Part model, mm, in its own coordinate system. A direction names the side the tool comes from. Give positions to 0.01 mm unless a question says otherwise; leave off trailing zeros. Write each loop counter-clockwise with the first axis right and the second up, starting at its lowest first coordinate (ties: lowest second). Pieces come first, ordered by that corner, then holes. Notation, with made-up numbers: M 53,29.5 L 101,29.5 A26 ccw 101,51.5 Z; hole C 42.25,-15.5 d9. An arc over 180 degrees is marked long. Answer as CSV lines item,"result". Start each with the question number.
1) Slice it at B-B, the plane x = 7.25. Give the cut face in (y, z), plus the area to 3 significant figures.
2) Wall check: line 1 along X through (y, z) = (-0.5, 5.5); line 2 along Y through (x, z) = (-3, 2.45); line 3 along Y through (x, z) = (7, 0.75). Give the ranges that are in metal, low to high. Write a range as from..to.
3) Slice it at A-A, the plane z = 24.5. Give the cut face in (x, y), plus the area to 3 significant figures.
4) Slice it at D-D, the plane y = 0. Give the number of separate pieces and of enclosed holes in the cut face, plus the area to 3 significant figures.
5) Pin check, flat tips, straight feed: pin 1 Ø11.5 at (x, y) = (-2, 2.5) entering from +Z; pin 2 Ø1 at (y, z) = (5.5, 25) entering from -X; pin 3 Ø10 at (x, z) = (-6, 29) entering from -Y. Stop position of each tip, or through.
6) Tool access for faces 1 (the cylindrical face through (6.25, 3.03, 1.52)), 2 (the cylindrical face through (11.7, 0.1, 14.5)): list every direction of +Z, -Z, +X, -X, +Y, -Y with a clear straight run to the whole face (end or side of a thin tool).
7) Mould opens along Y. For faces 3 (the cylindrical face through (12.06, -2.22, 16.85)), 4 (the flat face through (-12, 0, 33)) say: pulls with the +Y half, pulls with the -Y half, needs draft (parallel to the pull), parting line crosses it, or undercut.
8) Slice it at C-C, the plane x = 0. Give the cut face in (y, z), plus the area to 3 significant figures.
```python
from build123d import *
from build123d.topology import SkipClean

# Parameters (mm, degrees)
SKETCH1_R                           = 12.7
BOSS_EXTRUDE1_DEPTH                 = 3
SKETCH2_R                           = 0.75
CUT_EXTRUDE1_DEPTH                  = 3
BOSS_EXTRUDE2_DEPTH                 = 30
CUT_EXTRUDE2_REACH                  = 39.571
CUT_EXTRUDE2_END_RADIUS             = 12.7
SKETCH4_R                           = 2.5
CUT_EXTRUDE2_DIRECTION_2_REACH      = 39.571
CUT_EXTRUDE2_DIRECTION_2_END_RADIUS = 12.7


with BuildPart() as part:
    # Sketch1 → Boss-Extrude1 (new body)
    with BuildSketch(Plane.XY):
        Circle(SKETCH1_R)
    extrude(amount=BOSS_EXTRUDE1_DEPTH)

    # Sketch2 → Cut-Extrude1 (cut)
    with BuildSketch(Plane.XY.offset(3)):
        with Locations((0, 7)):
            Circle(SKETCH2_R)
        with Locations((-3, 7)):
            Circle(SKETCH2_R)
        with Locations((3, 7)):
            Circle(SKETCH2_R)
        with Locations((7, -3)):
            Circle(SKETCH2_R)
        with Locations((7, 0)):
            Circle(SKETCH2_R)
        with Locations((7, 3)):
            Circle(SKETCH2_R)
        with Locations((-3, -7)):
            Circle(SKETCH2_R)
        with Locations((0, -7)):
            Circle(SKETCH2_R)
        with Locations((3, -7)):
            Circle(SKETCH2_R)
        with Locations((-7, 3)):
            Circle(SKETCH2_R)
        with Locations((-7, 0)):
            Circle(SKETCH2_R)
        with Locations((-7, -3)):
            Circle(SKETCH2_R)
    extrude(amount=-CUT_EXTRUDE1_DEPTH, mode=Mode.SUBTRACT)

    # Sketch3 → Boss-Extrude2 (add)
    with SkipClean():  # the faces are left unmerged after this step: merging them gives an invalid solid
        with BuildSketch(Plane.XY.offset(3)):
            with BuildLine():
                Line((-8.980256121, 8.980256121), (-8.273149436, 8.273149436))
                ThreePointArc((-8.273149436, 8.273149436), (-11.700000136, 0), (-8.27314937, -8.27314937))
                Line((-8.27314937, -8.27314937), (-8.980256121, -8.980256121))
                ThreePointArc((-8.980256121, -8.980256121), (-12.7, 0), (-8.980256121, 8.980256121))
            make_face()
            with BuildLine():
                Line((8.980256121, 8.980256121), (8.273149436, 8.273149436))
                ThreePointArc((8.273149436, 8.273149436), (11.700000136, 0), (8.27314937, -8.27314937))
                Line((8.27314937, -8.27314937), (8.980256121, -8.980256121))
                ThreePointArc((8.980256121, -8.980256121), (12.7, 0), (8.980256121, 8.980256121))
            make_face()
        extrude(amount=BOSS_EXTRUDE2_DEPTH)

    # Cut-Extrude2: up to this cylinder (the profile starts inside it)
    with SkipClean():  # the faces are left unmerged after this step: merging them gives an invalid solid
        cut_extrude2_end = Plane(origin=(0, 0, 18), z_dir=(0, 0, -1)) * Cylinder(CUT_EXTRUDE2_END_RADIUS, 125.542, mode=Mode.PRIVATE)
        # Sketch4 → Cut-Extrude2 (cut, up to the surface)
        with BuildSketch(Plane(origin=(0, 0, 0), x_dir=(0, 0, -1), z_dir=(1, 0, 0)), mode=Mode.PRIVATE) as cut_extrude2_sk1:
            with Locations((-8, 0)):
                Circle(SKETCH4_R)
        cut_extrude2_tool1 = extrude(cut_extrude2_sk1.sketch, amount=-CUT_EXTRUDE2_REACH, mode=Mode.PRIVATE) & cut_extrude2_end
        add(cut_extrude2_tool1.solids().sort_by_distance((0, 0, 8))[0], mode=Mode.SUBTRACT)
        # Sketch4 → Cut-Extrude2 (cut, up to the surface)
        with BuildSketch(Plane(origin=(0, 0, 0), x_dir=(0, 0, -1), z_dir=(1, 0, 0)), mode=Mode.PRIVATE) as cut_extrude2_sk2:
            with Locations((-18, 0)):
                Circle(SKETCH4_R)
        cut_extrude2_tool2 = extrude(cut_extrude2_sk2.sketch, amount=-CUT_EXTRUDE2_REACH, mode=Mode.PRIVATE) & cut_extrude2_end
        add(cut_extrude2_tool2.solids().sort_by_distance((0, 0, 18))[0], mode=Mode.SUBTRACT)
        # Sketch4 → Cut-Extrude2 (cut, up to the surface)
        with BuildSketch(Plane(origin=(0, 0, 0), x_dir=(0, 0, -1), z_dir=(1, 0, 0)), mode=Mode.PRIVATE) as cut_extrude2_sk3:
            with Locations((-28, 0)):
                Circle(SKETCH4_R)
        cut_extrude2_tool3 = extrude(cut_extrude2_sk3.sketch, amount=-CUT_EXTRUDE2_REACH, mode=Mode.PRIVATE) & cut_extrude2_end
        add(cut_extrude2_tool3.solids().sort_by_distance((0, 0, 28))[0], mode=Mode.SUBTRACT)

    # Cut-Extrude2 direction 2: up to this cylinder (the profile starts inside it)
    with SkipClean():  # the faces are left unmerged after this step: merging them gives an invalid solid
        cut_extrude2_direction_2_end = Plane(origin=(0, 0, 18), z_dir=(0, 0, -1)) * Cylinder(CUT_EXTRUDE2_DIRECTION_2_END_RADIUS, 125.542, mode=Mode.PRIVATE)
        # Sketch4 → Cut-Extrude2 direction 2 (cut, up to the surface)
        with BuildSketch(Plane(origin=(0, 0, 0), x_dir=(0, 0, -1), z_dir=(1, 0, 0)), mode=Mode.PRIVATE) as cut_extrude2_direction_2_sk1:
            with Locations((-8, 0)):
                Circle(SKETCH4_R)
        cut_extrude2_direction_2_tool1 = extrude(cut_extrude2_direction_2_sk1.sketch, amount=CUT_EXTRUDE2_DIRECTION_2_REACH, mode=Mode.PRIVATE) & cut_extrude2_direction_2_end
        add(cut_extrude2_direction_2_tool1.solids().sort_by_distance((0, 0, 8))[0], mode=Mode.SUBTRACT)
        # Sketch4 → Cut-Extrude2 direction 2 (cut, up to the surface)
        with BuildSketch(Plane(origin=(0, 0, 0), x_dir=(0, 0, -1), z_dir=(1, 0, 0)), mode=Mode.PRIVATE) as cut_extrude2_direction_2_sk2:
            with Locations((-18, 0)):
                Circle(SKETCH4_R)
        cut_extrude2_direction_2_tool2 = extrude(cut_extrude2_direction_2_sk2.sketch, amount=CUT_EXTRUDE2_DIRECTION_2_REACH, mode=Mode.PRIVATE) & cut_extrude2_direction_2_end
        add(cut_extrude2_direction_2_tool2.solids().sort_by_distance((0, 0, 18))[0], mode=Mode.SUBTRACT)
        # Sketch4 → Cut-Extrude2 direction 2 (cut, up to the surface)
        with BuildSketch(Plane(origin=(0, 0, 0), x_dir=(0, 0, -1), z_dir=(1, 0, 0)), mode=Mode.PRIVATE) as cut_extrude2_direction_2_sk3:
            with Locations((-28, 0)):
                Circle(SKETCH4_R)
        cut_extrude2_direction_2_tool3 = extrude(cut_extrude2_direction_2_sk3.sketch, amount=CUT_EXTRUDE2_DIRECTION_2_REACH, mode=Mode.PRIVATE) & cut_extrude2_direction_2_end
        add(cut_extrude2_direction_2_tool3.solids().sort_by_distance((0, 0, 28))[0], mode=Mode.SUBTRACT)


solid = part.part
```
Found:
1,outline,"M -10.43,0 L -3.71,0 L -3.71,3 L -10.43,3 Z; M -2.29,0 L -0.71,0 L -0.71,3 L -2.29,3 Z; M 0.71,0 L 2.29,0 L 2.29,3 L 0.71,3 Z; M 3.71,0 L 10.43,0 L 10.43,3 L 3.71,3 Z"
1,area,"49.8 mm²"
2,line 1,"-12.69..-11.69, 11.69..12.69"
2,line 2,"-12.34..-7.75, -6.25..6.25, 7.75..12.34"
2,line 3,"-10.6..-3.75, -2.25..-0.75, 0.75..2.25, 3.75..10.6"
3,outline,"M -8.98,-8.98 L -8.27,-8.27 A11.7 cw -8.27,8.27 L -8.98,8.98 A12.7 ccw Z; M 8.27,-8.27 L 8.98,-8.98 A12.7 ccw 8.98,8.98 L 8.27,8.27 A11.7 cw Z"
3,area,"38.3 mm²"
4,separate pieces,"9"
4,enclosed holes,"0"
4,area,"97.2 mm²"
5,pin 1,"z = 3"
5,pin 2,"x = -11.67"
5,pin 3,"y = -8.98"
6,face 1,"+Z, -Z"
6,face 2,"+Z"
7,face 3,"undercut"
7,face 4,"needs draft"
8,outline,"M -12.7,0 L -7.75,0 L -7.75,3 L -12.7,3 Z; M -6.25,0 L 6.25,0 L 6.25,3 L -6.25,3 Z; M 7.75,0 L 12.7,0 L 12.7,3 L 7.75,3 Z"
8,area,"67.2 mm²"
